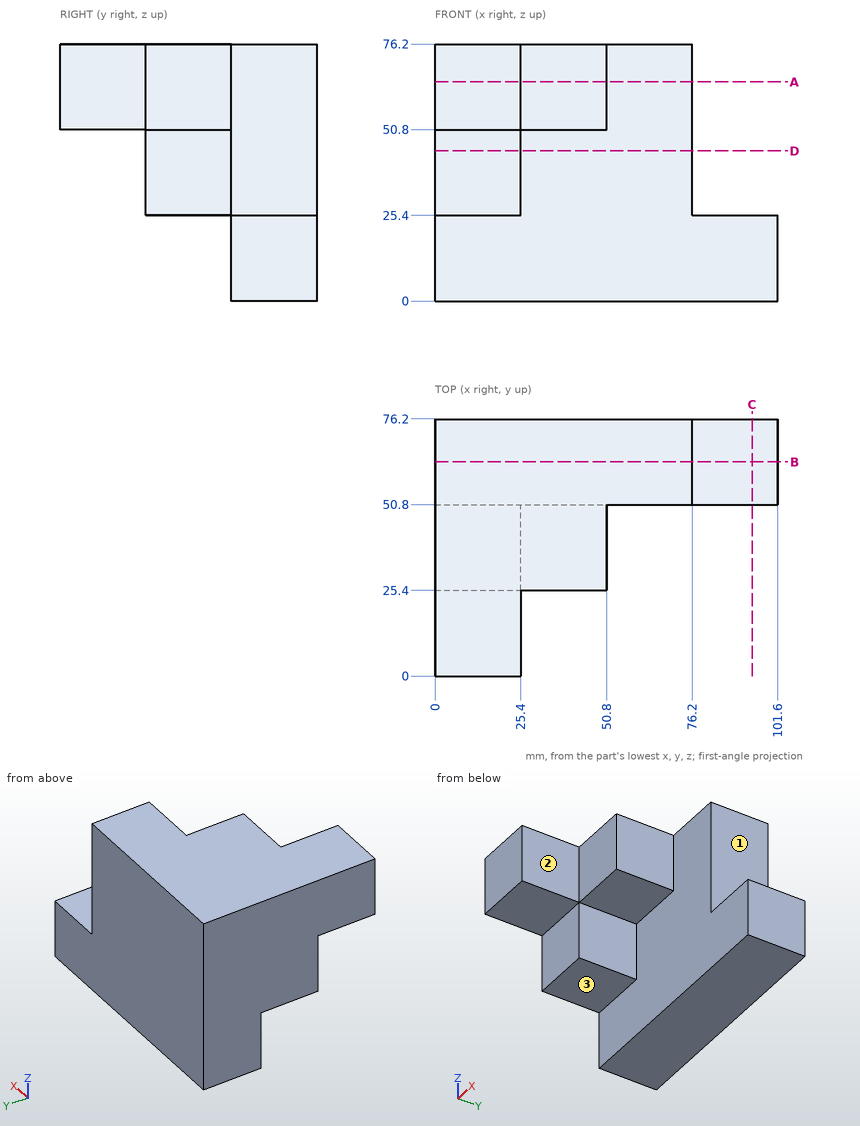
Geometry check sheet. Reference: drawing and pictorial views, mm from the part's lowest x, y, z. A direction names the side the tool comes from. Give positions to 0.01 mm unless a question says otherwise; leave off trailing zeros. Order: outer loops, then holes, each group sorted by start corner. A loop starts at its lowest first (then second) coordinate and runs counter-clockwise, first axis right, second up. Notation, with made-up numbers: M 24,43.5 L 80,43.5 A25 ccw 80,56.5 Z; hole C -28.75,-7 d6. An arc over 180 degrees is marked long. Use one line per item in the form item = value. Start each with the question number.
Q1. Section check C-C (x = 94). Enter the section's corners in (y, z).
Q2. Section check A-A (z = 65). Enter the section's corners in (x, y).
Q3. Section check B-B (y = 63.5). Enter the section's corners in (x, z), then the cut area to 3 significant figures.
Q4. Go/stop test with flat-tipped pins: pin 1 Ø4 at (x, z) = (73.5, 8) entering from -Y; pin 2 Ø12.5 at (y, z) = (35.5, 37.5) entering from +X; pin 3 Ø3 at (x, y) = (82, 51) entering from +Z. Record where each tip stops, or that it passes through.
Q5. Access from +Z, -Z, +X, -X, +Y, -Y to the whole of each face (thin tool, end or side, straight path). Record for the marked faces 1, 2 and 3.
Q6. Section check D-D (z = 44.5). Enter the section's corners in (x, y).
Q7. Scan lines: line 1 along Y through (x, z) = (64.5, 24); line 2 along Z through (x, y) = (11.5, 39.5). Record each from-to range of solid material in increasing order. Write a range as [from, to].
Evaluation:
q1.outline = M 50.8,0 L 76.2,0 L 76.2,25.4 L 50.8,25.4 Z
q2.outline = M 0,0 L 25.4,0 L 25.4,25.4 L 50.8,25.4 L 50.8,50.8 L 76.2,50.8 L 76.2,76.2 L 0,76.2 Z
q3.outline = M 0,0 L 101.6,0 L 101.6,25.4 L 76.2,25.4 L 76.2,76.2 L 0,76.2 Z
q3.area = 6,450 mm2
q4.pin_1 = 50.8
q4.pin_2 = 25.4
q4.pin_3 = 25.4
q5.face_1 = +Z, +X, +Y, -Y
q5.face_2 = +Z, -Z, +X, -Y
q5.face_3 = -Z, +X, -X, -Y
q6.outline = M 0,25.4 L 25.4,25.4 L 25.4,50.8 L 76.2,50.8 L 76.2,76.2 L 0,76.2 Z
q7.line_1 = [50.8, 76.2]
q7.line_2 = [25.4, 76.2]
